Could you check a few things on this model? Use its own coordinates, in mm. Give positions to 0.01 mm unless a question says otherwise; leave off trailing zeros. Write each loop counter-clockwise with the first axis right and the second up, starting at its lowest first coordinate (ties: lowest second). Pieces come first, ordered by that corner, then holes. Notation, with made-up numbers: M -37,-33.75 L -11,-33.75 A30 cw -11,-5.75 Z; hole C 77,43 d9. An arc over 180 degrees is marked long. Answer as a JSON object with one key per item and string values. Group by question number.
```python
from build123d import *

# Parameters (mm, degrees)
BOSS_EXTRUDE1_DEPTH = 491.49
SKETCH2_R           = 38.1
BOSS_EXTRUDE2_DEPTH = 304.8
SKETCH3_R           = 38.1
BOSS_EXTRUDE3_DEPTH = 304.8
SKETCH4_R           = 33.02
CUT_EXTRUDE1_DEPTH  = 1102.09


with BuildPart() as part:
    # Sketch1 → Boss-Extrude1 (new body)
    with BuildSketch(Plane(origin=(0, 0, 0), x_dir=(0, 0, -1), z_dir=(1, 0, 0))):
        with BuildLine():
            Line((27.94, 6.35), (27.94, -6.35))
            Line((27.94, -6.35), (37.567106623, -6.35))
            ThreePointArc((37.567106623, -6.35), (37.966542918, -3.186160517), (38.1, 0))
            ThreePointArc((38.1, 0), (37.966542918, 3.186160517), (37.567106623, 6.35))
            Line((37.567106623, 6.35), (27.94, 6.35))
        make_face()
        with BuildLine():
            Line((37.567106623, -6.35), (27.94, -6.35))
            Line((27.94, -6.35), (27.94, 6.35))
            Line((27.94, 6.35), (37.567106623, 6.35))
            ThreePointArc((37.567106623, 6.35), (-38.1, 0), (37.567106623, -6.35))
        make_face()
        with BuildLine():
            ThreePointArc((38.1, 0), (37.966542918, -3.186160517), (37.567106623, -6.35))
            Line((37.567106623, -6.35), (48.26, -6.35))
            Line((48.26, -6.35), (48.26, 6.35))
            Line((48.26, 6.35), (37.567106623, 6.35))
            ThreePointArc((37.567106623, 6.35), (37.966542918, 3.186160517), (38.1, 0))
        make_face()
    extrude(amount=-BOSS_EXTRUDE1_DEPTH)

    # Sketch2 → Boss-Extrude2 (add)
    with BuildSketch(Plane(origin=(0, 0, 0), x_dir=(0, 0, -1), z_dir=(1, 0, 0))):
        Circle(SKETCH2_R)
    extrude(amount=BOSS_EXTRUDE2_DEPTH)

    # Sketch3 → Boss-Extrude3 (add)
    with BuildSketch(Plane.ZY.offset(491.49)):
        Circle(SKETCH3_R)
    extrude(amount=BOSS_EXTRUDE3_DEPTH)

    # Sketch4 → Cut-Extrude1 (cut, through all)
    with BuildSketch(Plane.ZY.offset(796.29)):
        Circle(SKETCH4_R)
    extrude(amount=-CUT_EXTRUDE1_DEPTH, mode=Mode.SUBTRACT)


solid = part.part
```
1) If we section it at C-C, the plane y = -20: List the corners of the cut face in (x, z) for me, plus the area to 3 significant figures.
2) If we section it at B-B, the plane x = -115: List the corners of the cut face in (y, z) for me.
3) We'd pull the mould along Z, two halves only. Please class faces 1 (the flat face through (-796.29, 31.2, -11.5)), 2 (the cylindrical face through (-253.5, 9.9, 31.5)): released by +Z, released by -Z, zero draft, split by the parting line, or undercut.
4) I'm going to push flat-ended pins straight in: pin 1 (8 mm diameter, centred on y = 1, z = -31, fed in from +X); pin 2 (1.5 mm diameter, centred on x = -630.5, y = -28.5, fed in from -Z); pin 3 (10 mm diameter, centred on x = -461, y = -21.5, fed in from +Z); pin 4 (5.5 mm diameter, centred on x = -144.5, z = -45, fed in from -Y). Where does each tip first touch, or does it pass through?
5) Please list where these lines run through material, in increasing order: line 1 along Y through (x, z) = (-435, 0); line 2 along Z through (x, y) = (255, 1); line 3 along Y through (x, z) = (160, -22). Write a range as from..to.
6) If we section it at D-D, the plane x = 172.5: List the corners of the cut face in (y, z) for me, plus the area to 3 significant figures.
7) If we section it at A-A, the plane z = 0: List the corners of the cut face in (x, y) for me, plus the area to 3 significant figures.
Taken from the geometry:
{
 "1": {"outline": "M -796.29,-32.43 L 304.8,-32.43 L 304.8,-26.27 L -796.29,-26.27 Z; M -796.29,26.27 L 304.8,26.27 L 304.8,32.43 L -796.29,32.43 Z", "area": "13,600 mm²"},
 "2": {"outline": "M -6.35,-48.26 L 6.35,-48.26 L 6.35,-37.57 A38.1 ccw long -6.35,-37.57 Z; hole C 0,0 d66.04"},
 "3": {"face 1": "zero draft", "face 2": "undercut"},
 "4": {"pin 1": "x = 304.8", "pin 2": "z = -26.11", "pin 3": "z = 34.34", "pin 4": "y = -6.35"},
 "5": {"line 1": "-38.1..-33.02, 33.02..38.1", "line 2": "-38.09..-33, 33..38.09", "line 3": "-31.11..-24.62, 24.62..31.11"},
 "6": {"outline": "C 0,0 d76.2; hole C 0,0 d66.04", "area": "1,140 mm²"},
 "7": {"outline": "M -796.29,-38.1 L 304.8,-38.1 L 304.8,-33.02 L -796.29,-33.02 Z; M -796.29,33.02 L 304.8,33.02 L 304.8,38.1 L -796.29,38.1 Z", "area": "11,200 mm²"}
}
